Autodesk Inventor part; units mm, degrees
ref_plane "YZ Plane" through (0, 0, 0) normal (1, 0, 0) x (0, 1, 0)
ref_plane "XZ Plane" through (0, 0, 0) normal (0, 1, 0) x (-1, 0, 0)
ref_plane "XY Plane" through (0, 0, 0) normal (0, 0, 1) x (1, 0, 0)
sketch "Sketch1" plane through (0, 0, 0) normal (0, 1, 0) x (-1, 0, 0)
  line L0 (-7.5, -15) -> (7.5, -15)
  line L1 (7.5, -15) -> (7.5, 15)
  line L2 (7.5, 15) -> (-7.5, 15)
  line L3 (-7.5, 15) -> (-7.5, -15)
  line L4 (-7.5, -15) -> (7.5, 15) construction
  line L5 (7.5, -15) -> (-7.5, 15) construction
  point P0 (0, 0)
  dimension "d0" = 15
  dimension "d1" = 30
extrude "Extrusion1" add sketch "Sketch1" along normal blind 4
sketch "Sketch2" plane through (0, 4, 0) normal (0, 1, 0) x (1, 0, 0)
  line L0 (-7.5, 15) -> (-7.5, -15)
  line L1 (7.5, -15) -> (7.5, 15)
  line L2 (-7.5, 15) -> (7.5, 15)
  line L3 (7.5, 15) -> (7.5, 12.5)
  line L4 (7.5, 12.5) -> (-7.5, 12.5)
  line L5 (-7.5, 12.5) -> (-7.5, 15)
  line L6 (7.5, 0) -> (0, 0) construction
  line L7 (-7.5, -15) -> (-7.5, 15)
  line L8 (7.5, 15) -> (7.5, -15)
  line L9 (-7.5, -15) -> (7.5, -15)
  line L10 (7.5, -12.5) -> (-7.5, -12.5)
  point P0 (7.5, 15)
  point P1 (7.5, -15)
  point P2 (7.5, -12.5)
  dimension "d4" = 2.5
extrude "Extrusion2" add sketch "Sketch2" along normal blind 25 contours L2 L1 L4 L0 | L10 L1 L9 L0
sketch "Sketch4" plane through (7.5, 0, -15) normal (0, 0, -1) x (-1, 0, 0)
  line L0 (7.5, 0) -> (7.5, 7) construction
  line L1 (0, 0) -> (0, 29) construction
  line L2 (15, 4) -> (15, 29) construction
  line L3 (0, 4) -> (0, 29) construction
  line L4 (15, 7) -> (0, 7) construction
  line L5 (0, 29) -> (15, 29) construction
  line L6 (15, 29) -> (0, 7) construction
  line L7 (0, 29) -> (15, 7) construction
  circle A0 centre (7.5, 18) radius 6.5
  line L8 (7.5, 0) -> (7.5, 18) construction
  line L9 (15, 0) -> (0, 0) construction
  dimension "d12" = 7
  dimension "d13" = 13
  dimension "d14" = 34.287
extrude "Extrusion4" cut sketch "Sketch4" against normal blind 30
sketch "Sketch5" plane through (0, 0, 0) normal (0, -1, 0) x (1, 0, 0)
  line L0 (-7.5, 15) -> (7.5, 15) construction
  line L1 (-7.5, 15) -> (7.5, -15) construction
  line L2 (7.5, 15) -> (-7.5, -15) construction
  circle A0 centre (0, 0) radius 1.5
  dimension "d17" = 3
extrude "Extrusion5" cut sketch "Sketch5" against normal blind 5
properties part number "llanta_1"
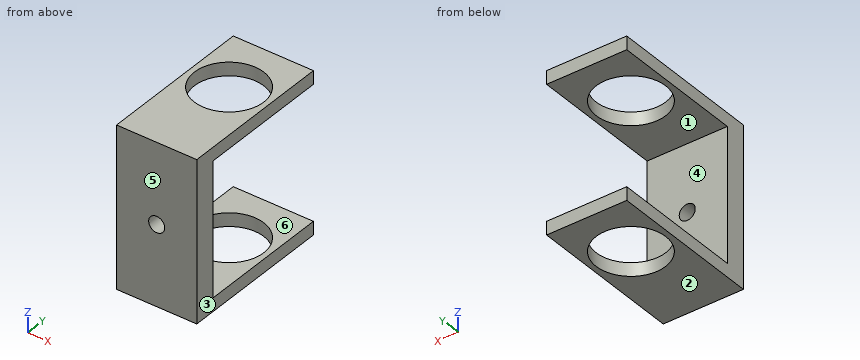
Could you check a few things on this model? Use its own coordinates, in mm. Face numbers are marked on the shaded views. A direction names the side the tool comes from. Round coordinates to 2 decimals unless told otherwise and drop trailing zeros. Loops run counter-clockwise (first coordinate to the right, second up) from the corner with the lowest first, then second, coordinate; pieces in that order, holes last. Notation, with made-up numbers: (-3.75, -36) -> (14.25, -36) arc R36 ccw to (14.25, 2) -> close; hole circle Ø1 at (79, 54). An arc over 180 degrees is marked (long way). Put each result on its own line as item: value.
Q1. I want a section at D-D on y = 18. Write out the boundary of the cut face in (x, z).
Checks:
outline: (-7.5, -15) -> (-6.5, -15) -> (-6.5, -12.5) -> (-7.5, -12.5) -> close; (-7.5, 12.5) -> (-6.5, 12.5) -> (-6.5, 15) -> (-7.5, 15) -> close; (6.5, -15) -> (7.5, -15) -> (7.5, -12.5) -> (6.5, -12.5) -> close; (6.5, 12.5) -> (7.5, 12.5) -> (7.5, 15) -> (6.5, 15) -> close
Q2. I want a section at C-C on x = -0.5. Write out the boundary of the cut face in (y, z), and give its area (3 significant figures).
Checks:
outline: (0, -15) -> (11.52, -15) -> (11.52, -12.5) -> (4, -12.5) -> (4, -1.41) -> (0, -1.41) -> close; (0, 1.41) -> (4, 1.41) -> (4, 12.5) -> (11.52, 12.5) -> (11.52, 15) -> (0, 15) -> close; (24.48, -15) -> (29, -15) -> (29, -12.5) -> (24.48, -12.5) -> close; (24.48, 12.5) -> (29, 12.5) -> (29, 15) -> (24.48, 15) -> close
area: 169 mm2
Q3. I want a section at A-A on z = 0. Write out the boundary of the cut face in (x, y), and give its area (3 significant figures).
Checks:
outline: (-7.5, 0) -> (-1.5, 0) -> (-1.5, 4) -> (-7.5, 4) -> close; (1.5, 0) -> (7.5, 0) -> (7.5, 4) -> (1.5, 4) -> close
area: 48.0 mm2
Q4. Thinking about a two-plate mould opening in Z: for the marked faces 1, 2, 3 and 4, which applies, pulls with the +Z half, pulls with the -Z half, needs draft (parallel to the pull), parting line crosses it, or undercut?
Checks:
face 1: undercut
face 2: pulls with the -Z half
face 3: needs draft
face 4: undercut
Q5. For pin 1 Ø8 at (x, z) = (1.5, 2) entering from +Y, with a flat end and sliding along its axis, tell me the tip position at first contact or that it passes through.
Checks:
pin 1: y = 4
Q6. Which directions (+Z, -Z, +X, -X, +Y, -Y) give clear straight access to the entire face, cutting with the end or side of a thin tool? Please do the marked faces 5 and 6.
Checks:
face 5: +Z, -Z, +X, -X, -Y
face 6: +X, -X, +Y
Q7. Please list where these lines run through material, in increasing order: line 1 (Y direction, x = 0, z = 13.6); line 2 (Z direction, x = -3, y = 9); line 3 (Z direction, x = 0, y = 1.75). Write a range as from..to.
Checks:
line 1: 0..11.5, 24.5..29
line 2: -15..-12.5, 12.5..15
line 3: -15..-1.5, 1.5..15
Q8. I want a section at B-B on y = 8.5. Write out the boundary of the cut face in (x, z).
Checks:
outline: (-7.5, -15) -> (7.5, -15) -> (7.5, -12.5) -> (-7.5, -12.5) -> close; (-7.5, 12.5) -> (7.5, 12.5) -> (7.5, 15) -> (-7.5, 15) -> close
